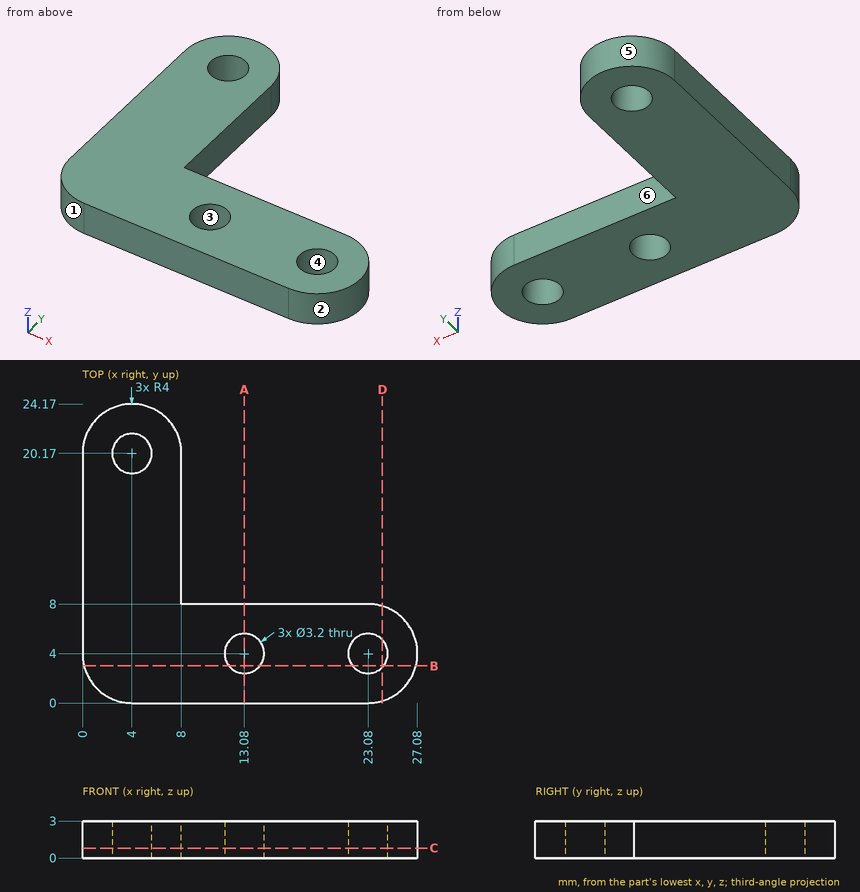
Here's the drawing with two shaded views (mm, measured from the low corner). I have some questions. A direction names the side the tool comes from. Coordinates: 2 decimals unless noted, no trailing zeros. Loops run counter-clockwise (first coordinate to the right, second up) from the corner with the lowest first, then second, coordinate; pieces in that order, holes last. Notation, with made-up numbers: (82.5, 22) -> (103.5, 22) arc R25 cw to (103.5, 54) -> close; hole circle Ø10 at (35.5, -2.75). An arc over 180 degrees is marked (long way). Put each result on its own line as item: value. Start each with the question number.
Q1. If I drill on line 1 (Y direction, x = 13.08, z = 0.8); line 2 (X direction, y = 4.25, z = 0.5); line 3 (Y direction, x = 4, z = 2), over which ranges is the centre line in solid material (lowest first)? Write a range as [from, to].
Q2. I want a section at A-A (x = 13.08). Write out the boundary of the cut face in (y, z), plus the area to 3 significant figures.
Q3. I want a section at C-C (z = 0.8). Write out the boundary of the cut face in (x, y), plus the area to 3 significant figures.
Q4. Thinking about a two-plate mould opening in Y: for the marked faces 1, 2, 3 and 4, which applies, pulls with the +Y half, pulls with the -Y half, needs draft (parallel to the pull), parting line crosses it, or undercut?
Q5. I want a section at B-B (y = 3). Write out the boundary of the cut face in (x, z), plus the area to 3 significant figures.
Q6. I want a section at D-D (x = 24.25). Write out the boundary of the cut face in (y, z), plus the area to 3 significant figures.
Q7. For the marked faces 5 and 6, which set-ups out of +Z, -Z, +X, -X, +Y, -Y let a thin tool reach every point of the face, with its end or its side?
Q8. I'm going to push flat-ended pins straight in: P1, Ø3, axis at x = 23.08, y = 4, coming from the -Z side; P2, Ø4, axis at x = 13.08, y = 4, coming from the -Z side; P3, Ø0.9, axis at y = 14, z = 2, coming from the +X side. Where does each tip first touch, or does it pass through?
Taken from the geometry:
1. line 1: y = [0, 2.4], [5.6, 8]
1. line 2: x = [0, 11.5], [14.66, 21.5], [24.66, 27.07]
1. line 3: y = [0, 18.57], [21.77, 24.17]
2. outline: (0, 0) -> (2.4, 0) -> (2.4, 3) -> (0, 3) -> close; (5.6, 0) -> (8, 0) -> (8, 3) -> (5.6, 3) -> close
2. area: 14.4 mm2
3. outline: (0, 4) arc R4 ccw to (4, 0) -> (23.08, 0) arc R4 ccw to (23.08, 8) -> (8, 8) -> (8, 20.17) arc R4 ccw to (0, 20.17) -> close; hole circle Ø3.2 at (4, 20.17); hole circle Ø3.2 at (13.08, 4); hole circle Ø3.2 at (23.08, 4)
3. area: 305 mm2
4. face 1: pulls with the -Y half
4. face 2: parting line crosses it
4. face 3: undercut
4. face 4: undercut
5. outline: (0.13, 0) -> (11.83, 0) -> (11.83, 3) -> (0.13, 3) -> close; (14.33, 0) -> (21.83, 0) -> (21.83, 3) -> (14.33, 3) -> close; (24.33, 0) -> (26.95, 0) -> (26.95, 3) -> (24.33, 3) -> close
5. area: 65.5 mm2
6. outline: (0.17, 0) -> (2.91, 0) -> (2.91, 3) -> (0.17, 3) -> close; (5.09, 0) -> (7.83, 0) -> (7.83, 3) -> (5.09, 3) -> close
6. area: 16.4 mm2
7. face 5: +Z, -Z, +Y
7. face 6: +Z, -Z, +X, +Y
8. P1: passes through
8. P2: stops at z = 0
8. P3: stops at x = 8
